```python
from build123d import *

# Parameters (mm, degrees)
SKETCH1_W               = 29
SKETCH1_H               = 20
BOSS_EXTRUDE1_DEPTH     = 7.5
SKETCH2_R               = 3.175
CUT_EXTRUDE1_DEPTH      = 26.816661287
FILLET2_R               = 7.5
CUT_EXTRUDE2_REACH      = 33.579
CUT_EXTRUDE2_END_RADIUS = 3.175
SKETCH3_R               = 3.175
FILLET3_R               = 5
FILLET4_R               = 1


with BuildPart() as part:
    # Sketch1 → Boss-Extrude1 (new, symmetric)
    with BuildSketch(Plane(origin=(0, 0, 0), x_dir=(1, 0, 0), z_dir=(0, 1, 0))):
        Rectangle(SKETCH1_W, SKETCH1_H)
    extrude(amount=BOSS_EXTRUDE1_DEPTH, both=True)

    # Sketch2 → Cut-Extrude1 (cut, through all)
    with BuildSketch(Plane.XY.offset(10)):
        with Locations((-7, 0)):
            Circle(SKETCH2_R)
    extrude(amount=-CUT_EXTRUDE1_DEPTH, mode=Mode.SUBTRACT)

    # Fillet2
    fillet2_edges = [part.edges().sort_by_distance(p)[0] for p in [
        (-14.5, 7.5, 0),
        (-14.5, -7.5, 0),
    ]]
    fillet(fillet2_edges, radius=FILLET2_R - 0.0001)  # a hair under: the kernel refuses the full size

    # Cut-Extrude2: up to this cylinder (the profile starts outside it)
    cut_extrude2_end = Plane(origin=(-7, 0, 0), z_dir=(0, 0, 1)) * Cylinder(CUT_EXTRUDE2_END_RADIUS, 74.508, mode=Mode.PRIVATE)
    # Sketch3 → Cut-Extrude2 (cut, up to the surface)
    with BuildSketch(Plane(origin=(14.5, 0, 0), x_dir=(0, 0, -1), z_dir=(1, 0, 0)), mode=Mode.PRIVATE) as cut_extrude2_sk1:
        Circle(SKETCH3_R)
    cut_extrude2_tool1 = extrude(cut_extrude2_sk1.sketch, amount=-CUT_EXTRUDE2_REACH, mode=Mode.PRIVATE) - cut_extrude2_end
    add(cut_extrude2_tool1.solids().sort_by_distance((14.5, 0, 0))[0], mode=Mode.SUBTRACT)

    # Fillet3
    fillet3_edges = [part.edges().sort_by_distance(p)[0] for p in [
        (14.5, 0, -10),
        (14.5, 0, 10),
    ]]
    fillet(fillet3_edges, radius=FILLET3_R)

    # Fillet4
    fillet4_edges = [part.edges().sort_by_distance(p)[0] for p in [
        (1.24995, 7.5, 10),
        (1.24995, -7.5, 10),
        (-12.303330148, -5.303330148, 10),
        (-12.303330148, 5.303330148, 10),
        (-12.303330148, -5.303330148, -10),
        (-12.303330148, 5.303330148, -10),
        (1.24995, 7.5, -10),
        (1.24995, -7.5, -10),
        (14.5, -7.5, 0),
        (13.035533906, -7.5, 8.535533906),
        (13.035533906, -7.5, -8.535533906),
        (14.5, 7.5, 0),
        (13.035533906, 7.5, 8.535533906),
        (13.035533906, 7.5, -8.535533906),
    ]]
    fillet(fillet4_edges, radius=FILLET4_R)


solid = part.part
```
Input: part model. Units: mm. Frame: model coordinates. Give positions to 0.01 mm unless a question says otherwise; leave off trailing zeros. Order: outer loops, then holes, each group sorted by start corner. A loop starts at its lowest first (then second) coordinate and runs counter-clockwise, first axis right, second up. Notation, with made-up numbers: M 76.5,59 L 114.5,59 A36 cw 114.5,95 Z; hole C 36,-9 d4. An arc over 180 degrees is marked long. Return JSON: item names as keys, results as strings.
1) Contact query for flat-ended pins moving along their axis: pin 1 (3 mm diameter, centred on y = 5.5, z = 4.5, fed in from -X); pin 2 (3 mm diameter, centred on x = -10.5, z = 7.5, fed in from -Y); pin 3 (1 mm diameter, centred on y = 5.5, z = -5, fed in from -X). Output: stop coordinate, or through.
Taken from the geometry:
{"pin 1": "stops at x = -13.34", "pin 2": "stops at y = -7.23", "pin 3": "stops at x = -12.59"}
2) Mould query, pull axis Y, two halves, no side actions, for faces 1 (the face through (3.9, 0.14, 3.17)), 2 (the face through (0, 0, -10)), 3 (the face through (14.215, 7.199, -0.07)), 4 (the face through (-10.17, 0.14, 0.14)). Classes: released by +Y, released by -Y, zero draft, split by the parting line, or undercut.
Taken from the geometry:
{"face 1": "undercut", "face 2": "zero draft", "face 3": "released by +Y", "face 4": "undercut"}
3) Line query: L1, parallel to Y at x = -7, z = 1 (3 decimals); L2, parallel to Z at x = 8.25, y = 0 (3 decimals); L3, parallel to Y at x = -4.5, z = 8.75. Output: solid intervals per line, ascending. Write a range as [from, to].
Taken from the geometry:
{"L1": "y = [-7.5, -3.175], [3.175, 7.5]", "L2": "z = [-10, -3.175], [3.175, 10]", "L3": "y = [-7.5, -1.96], [1.96, 7.5]"}
4) Section query D-D on x = -4.25. Output: boundary loops of the cut face in (y, z) (3 decimals).
Taken from the geometry:
{"outline": "M -7.5,-9 A1 ccw -6.5,-10 L -1.587,-10 L -1.587,-2.75 A3.175 cw -1.587,2.75 L -1.587,10 L -6.5,10 A1 ccw -7.5,9 Z; M 1.587,-10 L 6.5,-10 A1 ccw 7.5,-9 L 7.5,9 A1 ccw 6.5,10 L 1.587,10 L 1.587,2.75 A3.175 cw 1.587,-2.75 Z"}
5) Section query A-A on x = 4.25. Output: boundary loops of the cut face in (y, z) (3 decimals), and give its area (3 significant figures).
Taken from the geometry:
{"outline": "M -7.5,-9 A1 ccw -6.5,-10 L 6.5,-10 A1 ccw 7.5,-9 L 7.5,9 A1 ccw 6.5,10 L -6.5,10 A1 ccw -7.5,9 Z; hole C 0,0 d6.35", "area": "267 mm2"}
